Work out the finished part from the listing and answer in its coordinate system (mm). A direction names the side the tool comes from. Coordinates: 2 decimals unless noted, no trailing zeros. Loops run counter-clockwise (first coordinate to the right, second up) from the corner with the lowest first, then second, coordinate; pieces in that order, holes last. Notation, with made-up numbers: M 77.25,-35 L 102.25,-35 A17 cw 102.25,-3 Z; hole C -9,47 d3. An arc over 180 degrees is marked long. Write each question's results on one line, items separated by ' | '.
```python
from build123d import *

# Parameters (mm, degrees)
BOSS_EXTRUDE1_DEPTH     = 7.2
SKETCH2_R               = 1.825
CUT_EXTRUDE1_DEPTH      = 47.2
CUT_EXTRUDE3_DEPTH      = 5
CUT_EXTRUDE3_DEPTH_BACK = 5.5
SKETCH3_R               = 2.85
CUT_EXTRUDE4_DEPTH      = 20


with BuildPart() as part:
    # Sketch1 → Boss-Extrude1 (new body)
    with BuildSketch(Plane(origin=(0, 0, 0), x_dir=(1, 0, 0), z_dir=(0, 1, 0))):
        with BuildLine():
            Line((-19.175, 0), (-30, 0))
            ThreePointArc((-30, 0), (0, 30), (30, 0))
            Line((30, 0), (19.175, 0))
            ThreePointArc((19.175, 0), (0, 19.175), (-19.175, 0))
        make_face()
    extrude(amount=BOSS_EXTRUDE1_DEPTH)

    # Sketch2 → Cut-Extrude1 (cut)
    with BuildSketch(Plane.XY):
        with Locations((-24.5875, 3.6)):
            Circle(SKETCH2_R)
        with Locations((24.5875, 3.6)):
            Circle(SKETCH2_R)
    extrude(amount=-CUT_EXTRUDE1_DEPTH, mode=Mode.SUBTRACT)

    # Sketch3 → Cut-Extrude3 (cut, two sides: drawn at the far end of the back side and taken through both)
    with BuildSketch(Plane(origin=(0, 0, -16.445655164), x_dir=(0, -1, 0), z_dir=(0, 0, -1)).offset(-CUT_EXTRUDE3_DEPTH_BACK)):
        with Locations(Location((-3.6, 24.5875, 0), (0, 0, 270))):
            Circle(SKETCH3_R)
        with Locations(Location((-3.6, -24.5875, 0), (0, 0, 270))):
            Circle(SKETCH3_R)
    extrude(amount=CUT_EXTRUDE3_DEPTH + CUT_EXTRUDE3_DEPTH_BACK, mode=Mode.SUBTRACT)

    # Sketch4 → Cut-Extrude4 (cut)
    with BuildSketch(Plane(origin=(0, 0, -10.945655164), x_dir=(1, 0, 0), z_dir=(0, 0, -1))):
        with BuildLine():
            Line((-30, -0.75), (-30, -6.45))
            Line((-30, -6.45), (-24.5875, -6.45))
            ThreePointArc((-24.5875, -6.45), (-21.7375, -3.6), (-24.5875, -0.75))
            Line((-24.5875, -0.75), (-30, -0.75))
        make_face()
        with BuildLine():
            Line((30, -0.75), (30, -6.45))
            Line((30, -6.45), (24.5875, -6.45))
            ThreePointArc((24.5875, -6.45), (21.7375, -3.6), (24.5875, -0.75))
            Line((24.5875, -0.75), (30, -0.75))
        make_face()
    extrude(amount=CUT_EXTRUDE4_DEPTH, mode=Mode.SUBTRACT)


solid = part.part
```
1) Straight lines are drawn through the part: probe 1 along Y at (x, z) = (-22, -12); probe 2 along Z at (x, y) = (-26.5, 3.5); probe 3 along X at (y, z) = (4.5, -8). For each, find the intervals that lie inside material, in ascending order. Write a range as [from, to].
Check result:
probe 1: [0, 2.41], [4.79, 7.2] | probe 2: [-10.95, 0] | probe 3: [-28.91, -26.18], [-23, -17.43], [17.43, 23], [26.18, 28.91]
2) Given pin 1 Ø2 at (y, z) = (1.5, -12) entering from -X; pin 2 Ø4 at (x, y) = (-2.5, 4.5) entering from +Z; pin 3 Ø2 at (y, z) = (3, -24.5) entering from +X; pin 4 Ø8 at (x, z) = (6, -10.5) entering from +Y, each flat-ended and moving along its own axis, determine where each tip first touches the part or whether it passes through.
Check result:
pin 1: x = -27.77 | pin 2: z = -18.64 | pin 3: x = 18.65 | pin 4: through
3) Which of the six approach directions +Z, -Z, +X, -X, +Y, -Y give full straight-line access (tool end or side, diameter ignored) to faces 1 (the face through (-26, 6.45, -13)), 2 (the face through (-0.66, 3.55, -29.993)), 3 (the face through (26, 0.75, -13))?
Check result:
face 1: -Z, -X | face 2: -Z, +Y, -Y | face 3: -Z, +X
4) For a pull along Y with two mould halves and no side action, classify faces 4 (the face through (-22.847, 4.148, -5.396)), 5 (the face through (26, 2, 0)), 6 (the face through (0, 0, -22)) as released by +Y, released by -Y, zero draft, split by the parting line, or undercut.
Check result:
face 4: undercut | face 5: zero draft | face 6: released by -Y
5) Find section D-D, the plane x = 0. Give the vertices of the cut face in (y, z) (3 decimals), and give its area (3 significant figures).
Check result:
outline: M 0,-30 L 7.2,-30 L 7.2,-19.175 L 0,-19.175 Z | area: 77.9 mm^2
6) Find section A-A, the plane y = 3.6. Give the number of separate pieces and of enclosed holes in the cut face, and give its area (3 significant figures).
Check result:
separate pieces: 3 | enclosed holes: 0 | area: 687 mm^2
7) Find section C-C, the plane z = -12. Give the vertices of the cut face in (x, y), and give its area (3 significant figures).
Check result:
outline: M -27.5,0 L -14.96,0 L -14.96,7.2 L -27.5,7.2 L -27.5,6.45 L -24.59,6.45 A2.85 cw -24.59,0.75 L -27.5,0.75 Z; M 14.96,0 L 27.5,0 L 27.5,0.75 L 24.59,0.75 A2.85 cw 24.59,6.45 L 27.5,6.45 L 27.5,7.2 L 14.96,7.2 Z | area: 122 mm^2
